The listing builds one solid part. Answer for the finished solid, in the listing's coordinates (mm). A direction names the side the tool comes from. Coordinates: 2 decimals unless noted, no trailing zeros. Loops run counter-clockwise (first coordinate to the right, second up) from the corner with the lowest first, then second, coordinate; pieces in that order, holes last. Notation, with made-up numbers: (-3.75, -35.75) -> (34.25, -35.75) arc R29 ccw to (34.25, -1.75) -> close; hole circle Ø3 at (67, 26.25). An arc over 180 degrees is marked (long way). Answer in a Markdown table with one row per item.
```python
from build123d import *

# Parameters (mm, degrees)
SKETCH_1_W      = 100
SKETCH_1_H      = 100
EXTRUDE_1_DEPTH = 3
SKETCH_4_W      = 100
SKETCH_4_H      = 100
EXTRUDE_4_DEPTH = 33
FILLET_3_R      = 8
SKETCH_7_R      = 1.5
EXTRUDE_6_DEPTH = 33


with BuildPart() as part:
    # Эскиз1 → Бобышка-Вытянуть1 (new body)
    with BuildSketch(Plane(origin=(0, 0, 0), x_dir=(1, 0, 0), z_dir=(0, 1, 0))):
        with Locations((50, 50)):
            Rectangle(SKETCH_1_W, SKETCH_1_H)
    extrude(amount=EXTRUDE_1_DEPTH)

    # Эскиз4 → Бобышка-Вытянуть4 (add)
    with BuildSketch(Plane(origin=(0, 3, 0), x_dir=(1, 0, 0), z_dir=(0, 1, 0))):
        with Locations((50, 50)):
            Rectangle(SKETCH_4_W, SKETCH_4_H)
        with BuildLine():
            Line((97, 97), (3, 97))
            Line((3, 97), (3, 64))
            ThreePointArc((3, 64), (2.899494937, 62.585786438), (2.6, 61.2))
            ThreePointArc((2.6, 61.2), (1, 50), (2.6, 38.8))
            ThreePointArc((2.6, 38.8), (2.899494937, 37.414213562), (3, 36))
            Line((3, 36), (3, 3))
            Line((3, 3), (97, 3))
            Line((97, 3), (97, 38.33809621))
            ThreePointArc((97, 38.33809621), (97.143892394, 40.02840472), (97.571428571, 41.670068722))
            ThreePointArc((97.571428571, 41.670068722), (99, 50), (97.571428571, 58.329931278))
            ThreePointArc((97.571428571, 58.329931278), (97.143892394, 59.97159528), (97, 61.66190379))
            Line((97, 61.66190379), (97, 97))
        make_face(mode=Mode.SUBTRACT)
    extrude(amount=EXTRUDE_4_DEPTH)

    # Скругление3
    fillet_3_edges = [part.edges().sort_by_distance(p)[0] for p in [
        (0, 18, -100),
        (100, 18, -100),
        (100, 18, 0),
        (0, 18, 0),
    ]]
    fillet(fillet_3_edges, radius=FILLET_3_R)

    # Эскиз7 → Бобышка-Вытянуть6 (add)
    # profile 1 of 4: a face of its own
    with BuildSketch(Plane(origin=(0, 3, 0), x_dir=(1, 0, 0), z_dir=(0, 1, 0))):
        with BuildLine():
            Line((3, 89), (3, 97))
            Line((3, 97), (11, 97))
            Line((11, 97), (11, 93))
            ThreePointArc((11, 93), (9.828427125, 90.171572875), (7, 89))
            Line((7, 89), (3, 89))
        make_face()
        with Locations(Location((7, 93, 0), (0, 0, 270))):
            Circle(SKETCH_7_R, mode=Mode.SUBTRACT)
    # profile 2 of 4: a face of its own
    with BuildSketch(Plane(origin=(0, 3, 0), x_dir=(1, 0, 0), z_dir=(0, 1, 0))):
        with BuildLine():
            Line((89, 93), (89, 97))
            Line((89, 97), (97, 97))
            Line((97, 97), (97, 89))
            Line((97, 89), (93, 89))
            ThreePointArc((93, 89), (90.171572875, 90.171572875), (89, 93))
        make_face()
        with Locations(Location((93, 93, 0), (0, 0, 90))):
            Circle(SKETCH_7_R, mode=Mode.SUBTRACT)
    # profile 3 of 4: a face of its own
    with BuildSketch(Plane(origin=(0, 3, 0), x_dir=(1, 0, 0), z_dir=(0, 1, 0))):
        with BuildLine():
            Line((97, 11), (97, 3))
            Line((97, 3), (89, 3))
            Line((89, 3), (89, 7))
            ThreePointArc((89, 7), (90.171572875, 9.828427125), (93, 11))
            Line((93, 11), (97, 11))
        make_face()
        with Locations(Location((93, 7, 0), (0, 0, 270))):
            Circle(SKETCH_7_R, mode=Mode.SUBTRACT)
    # profile 4 of 4: a face of its own
    with BuildSketch(Plane(origin=(0, 3, 0), x_dir=(1, 0, 0), z_dir=(0, 1, 0))):
        with BuildLine():
            Line((11, 7), (11, 3))
            Line((11, 3), (3, 3))
            Line((3, 3), (3, 11))
            Line((3, 11), (7, 11))
            ThreePointArc((7, 11), (9.828427125, 9.828427125), (11, 7))
        make_face()
        with Locations(Location((7, 7, 0), (0, 0, 90))):
            Circle(SKETCH_7_R, mode=Mode.SUBTRACT)
    extrude(amount=EXTRUDE_6_DEPTH)


solid = part.part
```
Item 1: A cutting plane is placed at C-C, the plane y = 24.5. Count the separate pieces of the cut face and the enclosed holes in it, plus the area to 3 significant figures.
Findings below:
| item | result |
|---|---|
| separate pieces | 1 |
| enclosed holes | 5 |
| area | 1,260 mm2 |
Item 2: Find the intervals of material crossed by probe 1 along Z at (x, y) = (32.5, 7); probe 2 along X at (y, z) = (31, -32.5); probe 3 along X at (y, z) = (27, -7), in increasing order.
Findings below:
| item | result |
|---|---|
| probe 1 | z = -100 to -97, -3 to 0 |
| probe 2 | x = 0 to 3, 97 to 100 |
| probe 3 | x = 0.06 to 5.5, 8.5 to 11, 89 to 91.5, 94.5 to 99.94 |
Item 3: A cutting plane is placed at A-A, the plane z = -79.5. Determine the outline of the cut face in (x, y), plus the area to 3 significant figures.
Findings below:
| item | result |
|---|---|
| outline | (0, 0) -> (100, 0) -> (100, 36) -> (97, 36) -> (97, 3) -> (3, 3) -> (3, 36) -> (0, 36) -> close |
| area | 498 mm2 |
Item 4: Determine the mould class of faces 3 (the face through (7, 3, -93)), 4 (the face through (100, 18, -49)), 5 (the face through (49, 18, 0)) for opening direction X: +X half, -X half, draft (parallel to the pull), parting line (faces both ways), or undercut.
Findings below:
| item | result |
|---|---|
| face 3 | undercut |
| face 4 | +X half |
| face 5 | draft |
Item 5: A cutting plane is placed at B-B, the plane x = 80. Determine the outline of the cut face in (y, z).
Findings below:
| item | result |
|---|---|
| outline | (0, -100) -> (36, -100) -> (36, -97) -> (3, -97) -> (3, -3) -> (36, -3) -> (36, 0) -> (0, 0) -> close |
Item 6: Flat-ended cylindrical pins translate along their axes: pin 1 Ø2 at (y, z) = (27.5, -95) entering from -X; pin 2 Ø1.5 at (x, z) = (7.5, -93.5) entering from +Y; pin 3 Ø2 at (y, z) = (15, -4.5) entering from -X; pin 4 Ø4.5 at (x, y) = (94, 18.5) entering from +Z. Find the tip coordinate at first contact, or state that the pin passes through.
Findings below:
| item | result |
|---|---|
| pin 1 | stops at x = 0.25 |
| pin 2 | stops at y = 3 |
| pin 3 | stops at x = 0.4 |
| pin 4 | stops at z = 0 |
Item 7: A tool of negligible diameter and unlimited length cuts with its end or side. For faces 1 (the face through (2.9, 19.3, -37.4)), 2 (the face through (49, 18, -100)), from which of +Z, -Z, +X, -X, +Y, -Y can it reach the whole face along a straight path? Write none if from no direction.
Findings below:
| item | result |
|---|---|
| face 1 | +Y |
| face 2 | -Z, +X, -X, +Y, -Y |
